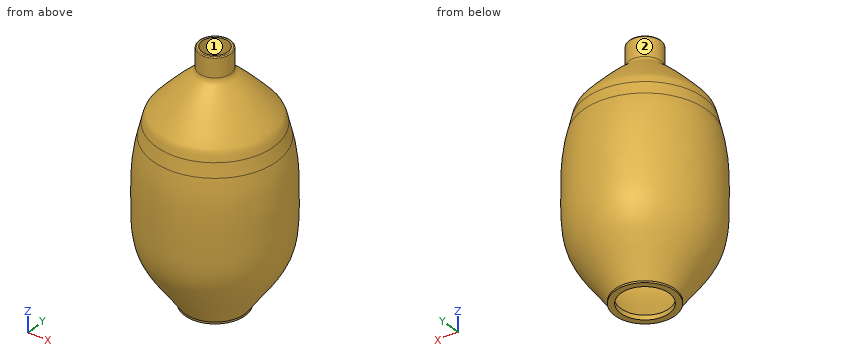
from build123d import *

# Parameters (mm, degrees)
FILLET1_R = 1
FILLET2_R = 261


with BuildPart() as part:
    # Sketch1 → Revolve1 (revolve)
    with BuildSketch(Plane(origin=(0, 0, 0), x_dir=(0, 0, -1), z_dir=(1, 0, 0)), mode=Mode.PRIVATE) as revolve1_sk:
        with BuildLine():
            Line((397.829689357, 442.030732016), (397.829689357, 437.465253038))
            Line((397.829689357, 437.465253038), (402.727304025, 437.465253038))
            Line((402.727304025, 437.465253038), (402.727304025, 443.706389044))
            Line((402.727304025, 443.706389044), (400.829689357, 443.706389044))
            add(Edge.make_bspline(
                [(225.76140421, 476.325643568), (250.097154316, 483.947478248), (288.266169539, 483.178078388), (352.940868229, 484.072298296), (383.102413409, 454.45631069), (400.829689357, 443.706389044)],
                knots=[0, 0, 0, 0, 0.382825495, 0.647952242, 1, 1, 1, 1], degree=3))
            add(Edge.make_bspline(
                [(161.570212669, 428.417840368), (165.387317703, 428.899023227), (168.912039636, 433.839023317), (180.956918186, 447.658310633), (194.029510768, 459.18780802), (209.789233312, 474.129612163), (219.574597702, 474.874030186), (225.76140421, 476.325643568)],
                knots=[0, 0, 0, 0, 0.12290588, 0.217110061, 0.671782411, 0.762907204, 1, 1, 1, 1], degree=3))
            Line((161.570212669, 428.417840368), (140.267729398, 428.417840368))
            Line((140.267729398, 428.417840368), (140.267729398, 425.417840368))
            Line((140.267729398, 425.417840368), (143.267729398, 425.417840368))
            Line((143.267729398, 425.417840368), (161.758556822, 425.417840368))
            add(Edge.make_bspline(
                [(161.758556822, 425.417840368), (161.819419658, 425.425512714), (161.923120579, 425.438145407), (162.27472043, 425.485106802), (162.818178628, 425.577931536), (163.912921631, 425.834440667), (165.908538221, 426.594243839), (168.218246537, 428.219309129), (170.253422656, 430.440677458), (171.873383547, 432.530119229), (173.443350782, 434.434741866), (175.634399053, 436.971222574), (178.464087021, 440.064030863), (181.967987343, 443.697716995), (185.564282324, 447.264008099), (189.237236912, 450.786660258), (192.970794515, 454.286260441), (196.748383607, 457.783072867), (199.920029625, 460.715970122), (202.461471471, 463.076565309), (204.3718093, 464.876742197), (206.193375261, 466.537080564), (207.988492092, 467.961738555), (209.784645287, 469.061554178), (211.812427443, 469.978689704), (214.014031173, 470.729433057), (217.153537993, 471.559261311), (221.356158221, 472.364854147), (224.841883019, 473.028424928), (226.55341987, 473.430003641)],
                knots=[-0.002005607, -0.002005607, -0.002005607, -0.002005607, -4.5902e-05, 0.001913803, 0.005833213, 0.013672034, 0.029349675, 0.060704958, 0.092060241, 0.123415523, 0.154770806, 0.186126089, 0.248836654, 0.311547219, 0.374257784, 0.436968349, 0.499678915, 0.56238948, 0.625100045, 0.656455328, 0.68781061, 0.719165893, 0.750521176, 0.781876458, 0.813231741, 0.844587023, 0.875942306, 0.938652871, 1.001363437, 1.001363437, 1.001363437, 1.001363437], degree=3))
            add(Edge.make_bspline(
                [(226.55341987, 473.430003641), (227.511334155, 473.730017583), (229.442395327, 474.313596579), (233.257020054, 475.370464775), (237.999385717, 476.518287604), (243.642274172, 477.63741249), (251.124673243, 478.823310695), (260.426034201, 479.796111148), (271.595398427, 480.356515998), (282.853796923, 480.523776333), (294.28732145, 480.496092928), (305.947870926, 480.5442697), (317.52750784, 480.329692321), (328.860803115, 479.392260986), (339.759791402, 477.348556138), (350.006050712, 473.722918078), (359.897969321, 468.470424151), (369.516520294, 462.162246785), (378.961959726, 455.277164683), (386.77531157, 449.497652391), (393.072202451, 445.099132849), (396.224580081, 443.034000768), (397.829689357, 442.030732016)],
                knots=[-0.000548601, -0.000548601, -0.000548601, -0.000548601, 0.014939032, 0.030426665, 0.061401931, 0.092377198, 0.123352464, 0.185302997, 0.24725353, 0.309204063, 0.371154595, 0.433105128, 0.495055661, 0.557006194, 0.618956726, 0.680907259, 0.742857792, 0.804808325, 0.866758858, 0.92870939, 0.959684657, 0.990659923, 0.990659923, 0.990659923, 0.990659923], degree=3))
        make_face()
    revolve(revolve1_sk.sketch.rotate(Axis((0, 411.495763099, -150.958062518), (0, 0, -1)), 90), axis=Axis((0, 411.495763099, -150.958062518), (0, 0, -1)))

    # Fillet1
    fillet1_edges = [part.edges().sort_by_distance(p)[0] for p in [
        (-16.922077268, 411.495763099, -140.267729398),
    ]]
    fillet(fillet1_edges, radius=FILLET1_R)

    # Fillet2
    # the kernel refuses this fillet: 261 mm, written as the material it adds along each edge
    with BuildSketch(Plane(origin=(0, 411.495763099, -225.76140421), x_dir=(1, 0, 0), z_dir=(0, 1, 0))) as fillet2_piece_1:
        with BuildLine():
            CenterArc((318.663368191, -61.563941431), FILLET2_R, 165.07684079, 3.104697334)
            Line((66.466358924, 5.649662228), (65.457570887, 5.918516643))
            ThreePointArc((65.457570887, 5.918516643), (64.675756472, 3.106461833), (63.833600693, 0.312029821))
            Line((63.833600693, 0.312029821), (63.813482761, 0.238477882))
            ThreePointArc((63.813482761, 0.238477882), (62.964491393, -3.853314586), (62.174322305, -7.894329204))
            Line((62.174322305, -7.894329204), (63.196191014, -8.10815236))
        make_face()
    revolve(axis=Axis((0, 411.495763099, -225.76140421), (0, 0, -1)))


solid = part.part
The model under review builds one solid part; all positions refer to its coordinate system, in mm. Face numbers are marked on the shaded views. Coordinates: 2 decimals unless noted, no trailing zeros. Answer in a Markdown table with one row per item.
(1) Insertion check: pin 1 (5 mm diameter, centred on x = -38, z = -264, fed in from -Y); pin 2 (4 mm diameter, centred on x = 22.5, y = 419, fed in from -Z); pin 3 (10 mm diameter, centred on x = 18, z = -330.5, fed in from -Y). Each pin has a flat end and moves straight along its axis. Give the tip position at first contact, or say it passes through.
Answers:
| item | result |
|---|---|
| pin 1 | y = 349.48 |
| pin 2 | z = -175.88 |
| pin 3 | y = 341.99 |
(2) The part is to be moulded in two halves that separate along X. For the marked faces 1 and 2, say which applies: +X half, -X half, draft (parallel to the pull), parting line (faces both ways), or undercut.
Answers:
| item | result |
|---|---|
| face 1 | undercut |
| face 2 | parting line |
(3) Wall thickness on line 1 along Y through (x, z) = (0, -156); line 2 along X through (y, z) = (394.5, -190.5); line 3 along Y through (x, z) = (0, -400): over which ranges is each line inside the solid? List them lowest first.
Answers:
| item | result |
|---|---|
| line 1 | 394.57 to 397.57, 425.42 to 428.42 |
| line 2 | -41.21 to -36.73, 36.73 to 41.21 |
| line 3 | 378.78 to 385.53, 437.47 to 444.21 |
